Autodesk Inventor part; units mm, degrees
ref_plane "YZ Plane" through (0, 0, 0) normal (1, 0, 0) x (0, 1, 0)
ref_plane "XZ Plane" through (0, 0, 0) normal (0, 1, 0) x (-1, 0, 0)
ref_plane "XY Plane" through (0, 0, 0) normal (0, 0, 1) x (1, 0, 0)
sketch "Sketch1" plane through (0, 0, 0) normal (0, 0, 1) x (1, 0, 0)
  line L0 (0, 0) -> (38.1, 0)
  line L1 (38.1, 0) -> (38.1, -184.15)
  line L2 (38.1, -184.15) -> (0, -184.15)
  line L3 (0, -184.15) -> (0, 0)
  dimension "d0" = 38.1
  dimension "d1" = 184.15
extrude "Extrusion1" add sketch "Sketch1" along normal blind 1764.792
sketch "Sketch2" plane through (38.1, -184.15, 0) normal (1, 0, 0) x (0, 0, -1)
  line L0 (0, 0) -> (-1764.792, 0)
  line L1 (-381, 0) -> (-381, 44.45)
  line L2 (-381, 44.45) -> (-304.8, 44.45)
  line L3 (-304.8, 44.45) -> (-304.8, 0)
  line L4 (0, 184.15) -> (0, 0)
  dimension "d4" = 44.45
  dimension "d5" = 76.2
  dimension "d6" = 304.8
extrude "Extrusion2" cut sketch "Sketch2" against normal through all
properties part number "Left End Board" material "Wood (Birch)"
Check sheet for the modelled part. Datum: model origin and axes. Units: mm. A direction names the side the tool comes from. Give positions to 0.01 mm unless a question says otherwise; leave off trailing zeros. Write each loop counter-clockwise with the first axis right and the second up, starting at its lowest first coordinate (ties: lowest second). Pieces come first, ordered by that corner, then holes.
Item 1: Draft check along Z on faces 1 (the face through (19, -91, 1764.792)), 2 (the face through (19, -91, 0)), 3 (the face through (19, -139.7, 343)). Enter one of: released by +Z, released by -Z, zero draft, split by the parting line, or undercut.
Item 2: Scan line: L1, parallel to Z at x = 12, y = -161. Record every from-to range of solid material in increasing order.
Item 3: Gauge pin test, flat end, axial feed: pin 1 (11.5 mm diameter, centred on x = 21, z = 358.5, fed in from -Y). Record the tip position at first contact, or that the pin passes through.
Item 4: Cross-section at A-A (z = 335.5). Enter the section's corners in (x, y), and give its area (3 significant figures).
Item 5: Access from +Z, -Z, +X, -X, +Y, -Y to the whole of each face (thin tool, end or side, straight path). Record for faces 4 (the face through (19, -184.15, 150)), 5 (the face through (19, -162, 304.8)).
Report:
1. face 1: released by +Z
1. face 2: released by -Z
1. face 3: undercut
2. L1: z = 0 to 304.8, 381 to 1764.79
3. pin 1: stops at y = -139.7
4. outline: (0, -139.7) - (38.1, -139.7) - (38.1, 0) - (0, 0) - close
4. area: 5,320 mm2
5. face 4: +Z, -Z, +X, -X, -Y
5. face 5: +X, -X, -Y
